```python
from build123d import *

# Parameters (mm, degrees)
F2_R     = 1
F3_DEPTH = 5
F4_R     = 11.019991
F5_DEPTH = 10


with BuildPart() as f1:
    # F0 (on Front) → F1 (revolve)
    with BuildSketch(Plane.XZ):
        Polygon((17.5, 0), (0, 0), (0, -13.5281), (11.019991, -13.5281), align=None)
    revolve(axis=Axis((0, 0, -6.76405), (0, 0, -1)))

    # F2 (on face) → F3 (cut)
    with BuildSketch(Plane.XY):
        with Locations((0, 12.5)):
            Circle(F2_R)
        with Locations((-12.5, 0)):
            Circle(F2_R)
        with Locations((12.5, 0)):
            Circle(F2_R)
        with Locations((0, -12.5)):
            Circle(F2_R)
    extrude(amount=-F3_DEPTH, mode=Mode.SUBTRACT)

    # F4 (on face) → F5 (join)
    with BuildSketch(Plane(origin=(0, 0, -13.5281), x_dir=(1, 0, 0), z_dir=(0, 0, -1))):
        Circle(F4_R)
    extrude(amount=F5_DEPTH)

    # F6 (on Front) → F7 (revolve)
    with BuildSketch(Plane.XZ):
        Polygon((0, -23.5281), (-11.019991, -23.5281), (-14, -33.603374), (0, -33.603374), align=None)
    revolve(axis=Axis((0, 0, -28.565737), (0, 0, -1)))


solid = f1.part
```
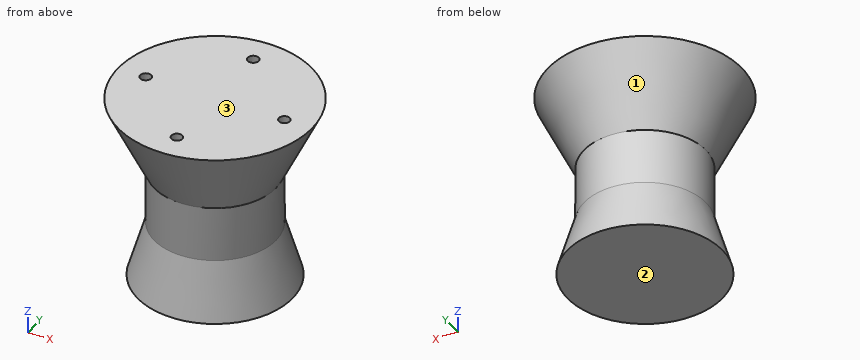
Read the model definition and answer for the solid it produces. Units are mm, in the model's axes. Face numbers are marked on the shaded views. Coordinates: 2 decimals unless noted, no trailing zeros. Order: outer loops, then holes, each group sorted by start corner. A loop starts at its lowest first (then second) coordinate and runs counter-clockwise, first axis right, second up. Notation, with made-up numbers: (40.25, 6) - (86.25, 6) arc R23 cw to (86.25, 26) - close; hole circle Ø2 at (3, 1). An arc over 180 degrees is marked (long way). Answer as a JSON object with one key per item and string values. Group by question number.
Item 1: Consider probe 1 along Y at (x, z) = (0, -1); probe 2 along Y at (x, z) = (0, -3); probe 3 along Z at (x, y) = (9.5, -10). Determine where each line is inside the solid, lowest interval first. Write a range as from..to.
Item 2: Section D-D (z = -9) is taken. Give the vertices of the cut face in (x, y), plus the area to 3 significant figures.
Item 3: Flat-ended cylindrical pins translate along their axes: P1, Ø8, axis at x = 5, z = -4.5, coming from the +Y side; P2, Ø1.8, axis at x = 0, y = 12.5, coming from the +Z side; P3, Ø4, axis at y = -12, z = -23, coming from the +X side. Find the tip coordinate at first contact, or state that the pin passes through.
Item 4: The mould has two halves that part along Z. Classify the marked faces 1, 2 and 3: +Z half, -Z half, draft (parallel to the pull), parting line (faces both ways), or undercut.
Item 5: Section C-C (z = -20.5) is taken. Give the vertices of the cut face in (x, y).
Item 6: Section A-A (x = 0) is taken. Give the vertices of the cut face in (y, z).
Results are:
{
 "1": {"probe 1": "y = -17.02..-13.5, -11.5..11.5, 13.5..17.02", "probe 2": "y = -16.06..-13.5, -11.5..11.5, 13.5..16.06", "probe 3": "z = -33.6..-32.9, -7.74..0"},
 "2": {"outline": "circle Ø26.38 at (0, 0)", "area": "546 mm^2"},
 "3": {"P1": "stops at y = 16.76", "P2": "stops at z = -5", "P3": "stops at x = 4.63"},
 "4": {"face 1": "undercut", "face 2": "-Z half", "face 3": "+Z half"},
 "5": {"outline": "circle Ø22.04 at (0, 0)"},
 "6": {"outline": "(-17.5, 0) - (-11.02, -13.53) - (-11.02, -23.53) - (-14, -33.6) - (14, -33.6) - (11.02, -23.53) - (11.02, -13.53) - (17.5, 0) - (13.5, 0) - (13.5, -5) - (11.5, -5) - (11.5, 0) - (-11.5, 0) - (-11.5, -5) - (-13.5, -5) - (-13.5, 0) - close"}
}
